from build123d import *

# Parameters (mm, degrees)
SKETCH1_W           = 25
SKETCH1_H           = 25
BOSS_EXTRUDE1_DEPTH = 7
SKETCH2_W           = 20
SKETCH2_H           = 20
CUT_EXTRUDE1_DEPTH  = 6
SKETCH3_R           = 1.25
BOSS_EXTRUDE2_DEPTH = 2
FILLET1_R           = 1
SKETCH4_R           = 1
BOSS_EXTRUDE3_DEPTH = 2


with BuildPart() as part:
    # Sketch1 → Boss-Extrude1 (new body)
    with BuildSketch(Plane(origin=(0, 0, 0), x_dir=(1, 0, 0), z_dir=(0, 1, 0))):
        Rectangle(SKETCH1_W, SKETCH1_H)
    extrude(amount=BOSS_EXTRUDE1_DEPTH)

    # Sketch2 → Cut-Extrude1 (cut)
    with BuildSketch(Plane(origin=(0, 7, 0), x_dir=(1, 0, 0), z_dir=(0, 1, 0))):
        Rectangle(SKETCH2_W, SKETCH2_H)
    extrude(amount=-CUT_EXTRUDE1_DEPTH, mode=Mode.SUBTRACT)

    # Sketch3 → Boss-Extrude2 (add)
    with BuildSketch(Plane(origin=(0, 1, 0), x_dir=(1, 0, 0), z_dir=(0, 1, 0))):
        Circle(SKETCH3_R)
    extrude(amount=BOSS_EXTRUDE2_DEPTH)

    # Fillet1
    fillet1_edges = [part.edges().sort_by_distance(p)[0] for p in [
        (-1.25, 3, 0),
    ]]
    fillet(fillet1_edges, radius=FILLET1_R)

    # Sketch4 → Boss-Extrude3 (add)
    with BuildSketch(Plane(origin=(0, 7, 0), x_dir=(1, 0, 0), z_dir=(0, 1, 0))):
        with Locations((-11, 11)):
            Circle(SKETCH4_R)
        with Locations((11, 11)):
            Circle(SKETCH4_R)
        with Locations((11, -11)):
            Circle(SKETCH4_R)
        with Locations((-11, -11)):
            Circle(SKETCH4_R)
    extrude(amount=BOSS_EXTRUDE3_DEPTH)


solid = part.part
Here's how the part is built. I have some questions about the finished solid (model axes, mm). A direction names the side the tool comes from. Give positions to 0.01 mm unless a question says otherwise; leave off trailing zeros. Order: outer loops, then holes, each group sorted by start corner. A loop starts at its lowest first (then second) coordinate and runs counter-clockwise, first axis right, second up. Notation, with made-up numbers: M 29,38 L 83,38 A26 ccw 83,60 Z; hole C 50,-26 d9. An arc over 180 degrees is marked long. Answer as a JSON object with one key per item and string values. Group by question number.
1) Please list where these lines run through material, in increasing order: L1, parallel to X at y = 5, z = 1; L2, parallel to Y at x = -2, z = 10.5. Write a range as [from, to].
2) Suppose I cut it at B-B, the plane y = 3.5. Write out the boundary of the cut face in (x, z).
3) Suppose I cut it at A-A, the plane x = 3.5. Write out the boundary of the cut face in (y, z).
4) On a 3-axis mill with a long thin cutter (end or side, diameter ignored), from which of +Z, -Z, +X, -X, +Y, -Y can I reach the whole of each face in a straight line? I mean faces 4 (the flat face through (-12.5, 3, 0)), 5 (the flat face through (-0.1, 7, -10.2)). Say none if no direction works.
5) We'd pull the mould along X, two halves only. Please class faces 1 (the flat face through (0, 3, 12.5)), 2 (the flat face through (12.5, 3, 0)), 3 (the flat face through (2, 1, 0)): pulls with the +X half, pulls with the -X half, needs draft (parallel to the pull), parting line crosses it, or undercut.
6) I'm going to push flat-ended pins straight in: pin 1 Ø2 at (x, z) = (-4.5, 1.5) entering from +Y; pin 2 Ø8 at (x, z) = (-6, -8) entering from +Y. Where does each tip first touch, or does it pass through?
7) Suppose I cut it at C-C, the plane z = -5.5. Write out the boundary of the cut face in (x, y).
8) Suppose I cut it at D-D, the plane z = 11. Write out the boundary of the cut face in (x, y), plus the area to 3 significant figures.
Results found:
{
 "1": {"L1": "[-12.5, -10], [10, 12.5]", "L2": "[0, 7]"},
 "2": {"outline": "M -12.5,-12.5 L 12.5,-12.5 L 12.5,12.5 L -12.5,12.5 Z; hole M -10,-10 L 10,-10 L 10,10 L -10,10 Z"},
 "3": {"outline": "M 0,-12.5 L 7,-12.5 L 7,-10 L 1,-10 L 1,10 L 7,10 L 7,12.5 L 0,12.5 Z"},
 "4": {"face 4": "+Z, -Z, -X, +Y, -Y", "face 5": "+Y"},
 "5": {"face 1": "needs draft", "face 2": "pulls with the +X half", "face 3": "undercut"},
 "6": {"pin 1": "y = 1", "pin 2": "y = 7"},
 "7": {"outline": "M -12.5,0 L 12.5,0 L 12.5,7 L 10,7 L 10,1 L -10,1 L -10,7 L -12.5,7 Z"},
 "8": {"outline": "M -12.5,0 L 12.5,0 L 12.5,7 L 12,7 L 12,9 L 10,9 L 10,7 L -10,7 L -10,9 L -12,9 L -12,7 L -12.5,7 Z", "area": "183 mm²"}
}
